Source: CAD feature listing. Evaluate the final solid. Frame: model axes, mm. Face numbers are marked on the shaded views. A direction names the side the tool comes from. Round coordinates to 2 decimals unless told otherwise and drop trailing zeros. Order: outer loops, then holes, each group sorted by start corner. A loop starts at its lowest first (then second) coordinate and runs counter-clockwise, first axis right, second up. Notation, with made-up numbers: (-24, -18.5) -> (11, -18.5) arc R14 ccw to (11, -13.5) -> close; hole circle Ø4 at (-35, 11.5). An arc over 180 degrees is marked (long way). Answer as CSV lines item,"result".
from build123d import *

# Parameters (mm, degrees)
F1_DEPTH = 63.5
F2_DEPTH = 25.4
F0_W     = 27.8559744183
F0_H     = 4.7498
F0_H_2   = 19.05
F3_DEPTH = 38.1
F4_DEPTH = 25.4
F6_R     = 5.08


with BuildPart() as f1:
    # F0 (on Front) → F1 (new body, symmetric)
    with BuildSketch(Plane.XZ):
        Polygon((-41.275, 9.525), (-41.275, -9.525), (41.275, -9.525), (41.275, 9.525), (22.225, 9.525), align=None)
    extrude(amount=F1_DEPTH, both=True)

    # F0 (on Front) → F2 (join, symmetric)
    with BuildSketch(Plane.XZ):
        with BuildLine():
            add(Edge.make_bspline(
                [(-41.275, 9.525), (-19.7094231844, 46.5213470161), (14.027427882, 62.8570914268), (57.15, 61.9252)],
                knots=[0, 0, 0, 0, 111.5045361635, 111.5045361635, 111.5045361635, 111.5045361635], degree=3))
            Line((-41.275, 9.525), (22.225, 9.525))
            Line((22.225, 9.525), (22.225, 27.0002))
            ThreePointArc((22.225, 27.0002), (32.4542956671, 51.6959043329), (57.15, 61.9252))
        make_face()
    extrude(amount=F2_DEPTH, both=True)

    # F0 (on Front) → F3 (join, symmetric)
    with BuildSketch(Plane.XZ):
        Polygon((85.725, 42.8752), (57.8690255817, 42.8752), (57.8690255817, 38.1), (108.6690255817, 38.1), (108.6690255817, 66.675), (85.725, 66.675), (85.725, 61.9252), align=None)
        with BuildLine():
            Line((22.225, 9.525), (41.275, 9.525))
            Line((41.275, 9.525), (41.275, 27.0002))
            ThreePointArc((41.275, 27.0002), (45.9246798487, 38.2255201513), (57.15, 42.8752))
            Line((57.15, 42.8752), (57.8690255817, 42.8752))
            Line((57.8690255817, 42.8752), (57.8690255817, 61.9252))
            Line((57.8690255817, 61.9252), (57.15, 61.9252))
            ThreePointArc((57.15, 61.9252), (32.4542956671, 51.6959043329), (22.225, 27.0002))
            Line((22.225, 27.0002), (22.225, 9.525))
        make_face()
        with Locations((71.7970127909, 64.3001)):
            Rectangle(F0_W, F0_H)
        with Locations((71.7970127909, 52.4002)):
            Rectangle(F0_W, F0_H_2)
    extrude(amount=F3_DEPTH, both=True)

    # F0 (on Front) → F4 (join)
    with BuildSketch(Plane.XZ):
        Polygon((-41.275, 9.525), (-41.275, -9.525), (41.275, -9.525), (41.275, 9.525), (22.225, 9.525), align=None)
        with BuildLine():
            add(Edge.make_bspline(
                [(-41.275, 9.525), (-19.7094231844, 46.5213470161), (14.027427882, 62.8570914268), (57.15, 61.9252)],
                knots=[0, 0, 0, 0, 111.5045361635, 111.5045361635, 111.5045361635, 111.5045361635], degree=3))
            Line((-41.275, 9.525), (22.225, 9.525))
            Line((22.225, 9.525), (22.225, 27.0002))
            ThreePointArc((22.225, 27.0002), (32.4542956671, 51.6959043329), (57.15, 61.9252))
        make_face()
        with BuildLine():
            Line((22.225, 9.525), (41.275, 9.525))
            Line((41.275, 9.525), (41.275, 27.0002))
            ThreePointArc((41.275, 27.0002), (45.9246798487, 38.2255201513), (57.15, 42.8752))
            Line((57.15, 42.8752), (57.8690255817, 42.8752))
            Line((57.8690255817, 42.8752), (57.8690255817, 61.9252))
            Line((57.8690255817, 61.9252), (57.15, 61.9252))
            ThreePointArc((57.15, 61.9252), (32.4542956671, 51.6959043329), (22.225, 27.0002))
            Line((22.225, 27.0002), (22.225, 9.525))
        make_face()
        with Locations((71.7970127909, 52.4002)):
            Rectangle(F0_W, F0_H_2)
        with Locations((71.7970127909, 64.3001)):
            Rectangle(F0_W, F0_H)
        Polygon((85.725, 42.8752), (57.8690255817, 42.8752), (57.8690255817, 38.1), (108.6690255817, 38.1), (108.6690255817, 66.675), (85.725, 66.675), (85.725, 61.9252), align=None)
    extrude(amount=F4_DEPTH)

    # F0 (on Front) → F5 (revolve)
    with BuildSketch(Plane.XZ):
        Polygon((85.725, 42.8752), (57.8690255817, 42.8752), (57.8690255817, 38.1), (108.6690255817, 38.1), (108.6690255817, 66.675), (85.725, 66.675), (85.725, 61.9252), align=None)
    revolve(axis=Axis((108.6690255817, 0, 52.3875), (0, 0, 1)))

    # F6
    f6_edges = [f1.edges().sort_by_distance(p)[0] for p in [
        (-41.275, 63.5, 0),
        (41.275, 63.5, 0),
        (-41.275, -63.5, 0),
        (41.275, -63.5, 0),
    ]]
    fillet(f6_edges, radius=F6_R)


solid = f1.part
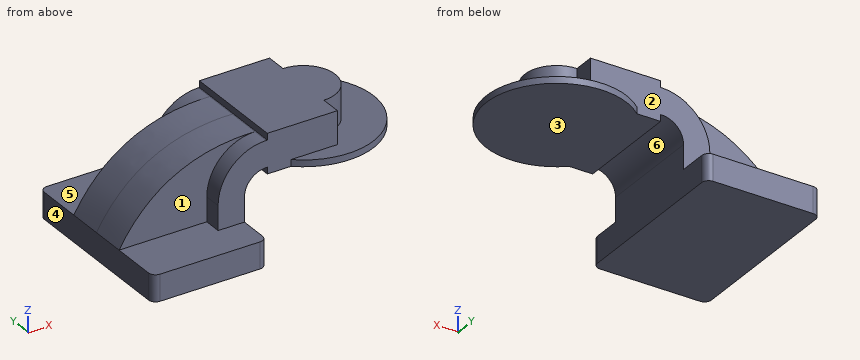
1. Reachability of the marked faces 1, 2 and 3 from +Z, -Z, +X, -X, +Y, -Y: full face, straight path, thin tool, end or side. Return the list, or none.
Results below:
face 1,"+Z, -X, -Y"
face 2,"+Z, -X, +Y"
face 3,"-Z, +X, +Y, -Y"
2. Section query B-B on x = 90. Return loops of the section in (y, z) (3 decimals).
Results below:
outline,"(-47.245, 38.1) -> (47.245, 38.1) -> (47.245, 42.875) -> (38.1, 42.875) -> (38.1, 66.675) -> (-38.1, 66.675) -> (-38.1, 42.875) -> (-47.245, 42.875) -> close"
3. Line query: L1, parallel to Z at x = 16, y = -34 (3 decimals); L2, parallel to X at y = 44, z = 0.5 (3 decimals); L3, parallel to X at y = -28, z = 19.5 (3 decimals). Output: solid intervals per line, ascending. Write a range as [from, to].
Results below:
L1,"[-9.525, 9.525]"
L2,"[-41.275, 41.275]"
L3,"[22.225, 41.275]"
4. Section query C-C on x = 146.5. Return loops of the section in (y, z).
Results below:
outline,"(-33.9, 38.1) -> (33.9, 38.1) -> (33.9, 42.88) -> (-33.9, 42.88) -> close"
5. Section query A-A on y = -46. Return loops of the section in (x, z) (3 decimals), and give its area (3 significant figures).
Results below:
outline,"(-41.275, -9.525) -> (41.275, -9.525) -> (41.275, 9.525) -> (-41.275, 9.525) -> close; (87.114, 38.1) -> (130.225, 38.1) -> (130.225, 42.875) -> (87.114, 42.875) -> close"
area,"1,780 mm2"
6. Mould query, pull axis X, two halves, no side actions, for the marked faces 4, 5 and 6. Classes: released by +X, released by -X, zero draft, split by the parting line, or undercut.
Results below:
face 4,"released by -X"
face 5,"zero draft"
face 6,"undercut"
7. Pin query (flat end, axial travel): pin 1 (6 mm diameter, centred on x = 107.5, y = 1, fed in from -Z); pin 2 (2 mm diameter, centred on y = 25, z = 9, fed in from +X) (3 decimals); pin 3 (1.5 mm diameter, centred on x = 87, y = 41, fed in from +Z); pin 4 (10 mm diameter, centred on y = 32, z = 14, fed in from -X) (3 decimals). Return the tip coordinate at first contact, or that it passes through.
Results below:
pin 1,"z = 38.1"
pin 2,"x = 41.275"
pin 3,"z = 42.88"
pin 4,"x = -41.275"
